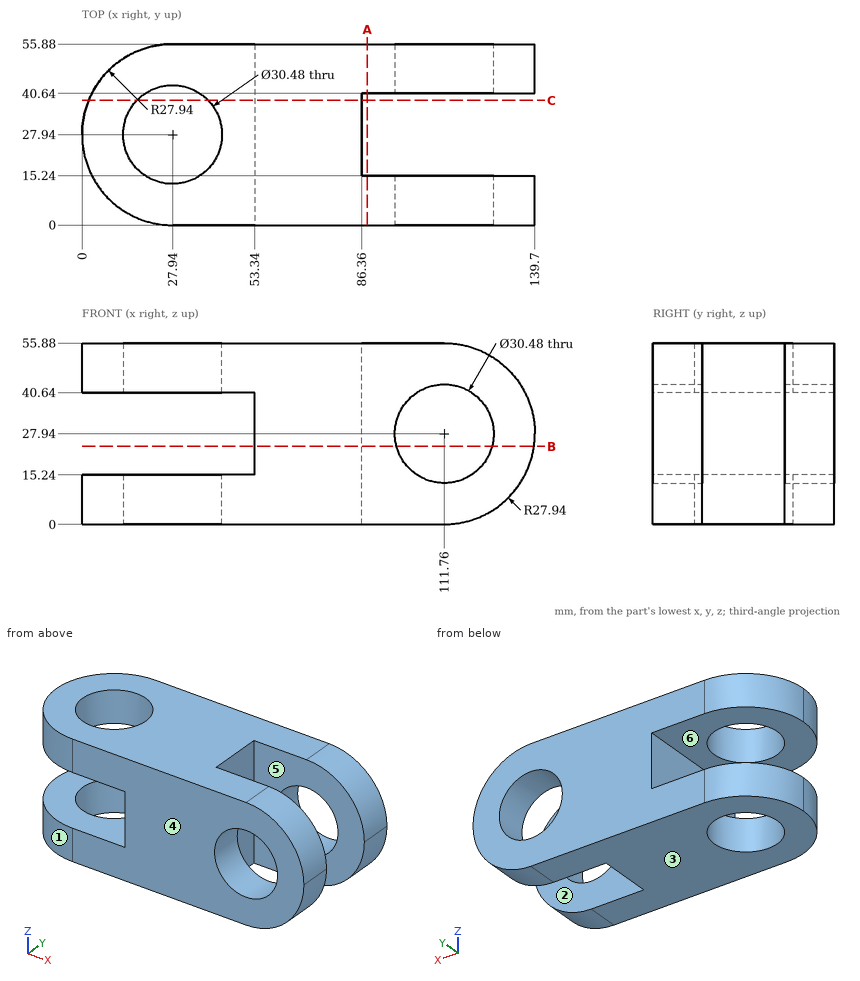
Source: three-view drawing plus pictorial views. Frame: mm from the lowest corner of the part. A direction names the side the tool comes from. Coordinates: 2 decimals unless noted, no trailing zeros. Order: outer loops, then holes, each group sorted by start corner. A loop starts at its lowest first (then second) coordinate and runs counter-clockwise, first axis right, second up. Notation, with made-up numbers: M 87.5,-9 L 133.5,-9 A24 cw 133.5,3 Z; hole C 68.25,-36.5 d5. An arc over 180 degrees is marked long. Write each question's results on one line, items separated by ' | '. Start each with the question number.
1. Reachability of the marked faces 4, 5 and 6 from +Z, -Z, +X, -X, +Y, -Y: full face, straight path, thin tool, end or side. Return the list, or none.
2. Material intervals for L1, parallel to X at y = 27, z = 42.5; L2, parallel to Y at x = 88, z = 43, sorted ascending.
3. Section A-A, the plane x = 88. Return the cut outline in (y, z).
4. Pin query (flat end, axial travel): pin 1 (20.5 mm diameter, centred on y = 32, z = 26.5, fed in from -X); pin 2 (3 mm diameter, centred on x = 121.5, z = 35.5, fed in from -Y); pin 3 (3 mm diameter, centred on y = 10.5, z = 47, fed in from -X); pin 4 (10 mm diameter, centred on y = 35.5, z = 18.5, fed in from +X). Return the tip coordinate at first contact, or that it passes through.
5. Section C-C, the plane y = 38.5. Return the cut outline in (x, z).
6. Draft query along Y for the marked faces 1, 2 and 3. Return one class per face: +Y half, -Y half, draft (parallel to the pull), parting line (faces both ways), or undercut.
7. Section B-B, the plane z = 24. Return the cut outline in (x, y).
Solution:
1) face 4: +Z, -Z, +X, -X, -Y | face 5: +Z, -Z, +X | face 6: -X, +Y, -Y
2) L1: 0.02 to 12.73, 43.15 to 86.36 | L2: 0 to 15.24, 40.64 to 55.88
3) outline: M 0,0 L 15.24,0 L 15.24,55.88 L 0,55.88 Z; M 40.64,0 L 55.88,0 L 55.88,55.88 L 40.64,55.88 Z
4) pin 1: x = 53.34 | pin 2: through | pin 3: x = 4.99 | pin 4: x = 86.36
5) outline: M 2.07,0 L 16.95,0 L 16.95,15.24 L 2.07,15.24 Z; M 2.07,40.64 L 16.95,40.64 L 16.95,55.88 L 2.07,55.88 Z; M 38.93,0 L 86.36,0 L 86.36,55.88 L 38.93,55.88 L 38.93,40.64 L 53.34,40.64 L 53.34,15.24 L 38.93,15.24 Z
6) face 1: -Y half | face 2: undercut | face 3: draft
7) outline: M 53.34,0 L 97.04,0 L 97.04,15.24 L 86.36,15.24 L 86.36,40.64 L 97.04,40.64 L 97.04,55.88 L 53.34,55.88 Z; M 126.48,0 L 139.42,0 L 139.42,15.24 L 126.48,15.24 Z; M 126.48,40.64 L 139.42,40.64 L 139.42,55.88 L 126.48,55.88 Z
